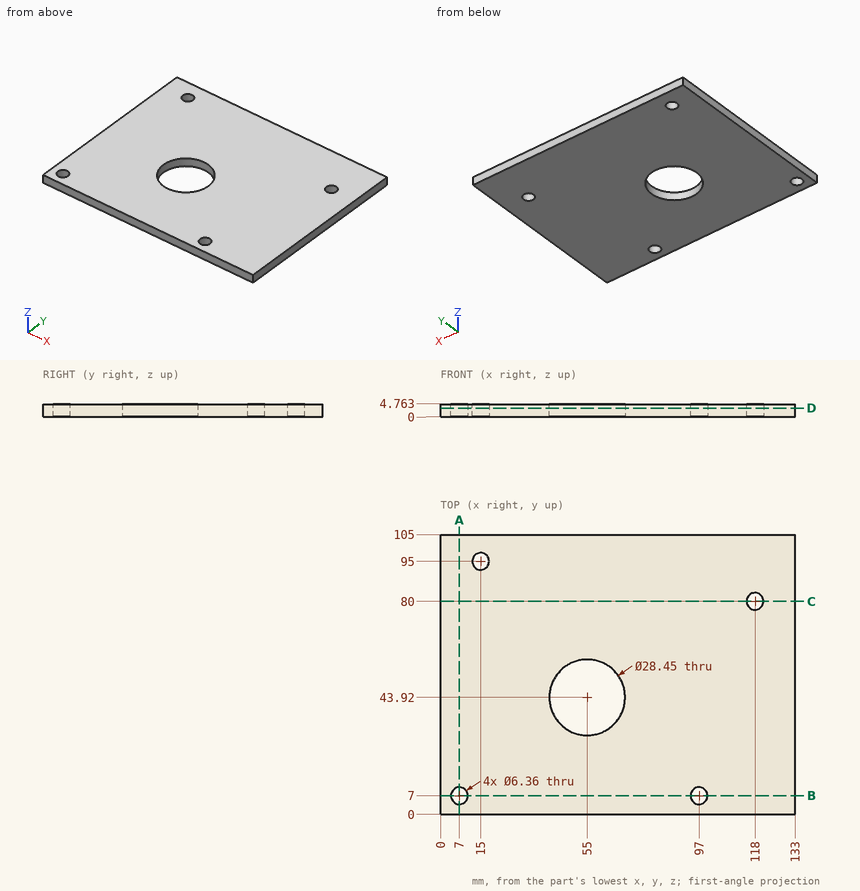
Geometry check sheet. Reference: drawing and pictorial views, mm from the part's lowest x, y, z. Give positions to 0.01 mm unless a question says otherwise; leave off trailing zeros. Order: outer loops, then holes, each group sorted by start corner. A loop starts at its lowest first (then second) coordinate and runs counter-clockwise, first axis right, second up. Notation, with made-up numbers: M -23.75,-16 L -8.75,-16 A23 ccw -8.75,19 Z; hole C 21,17 d7. An arc over 180 degrees is marked long. Answer in a Markdown table with one row per item.
1) Cross-section at A-A, the plane x = 7. Enter the section's corners in (y, z).
Filled sheet:
| item | result |
|---|---|
| outline | M 0,0 L 3.82,0 L 3.82,4.76 L 0,4.76 Z; M 10.18,0 L 105,0 L 105,4.76 L 10.18,4.76 Z |
2) Cross-section at C-C, the plane y = 80. Enter the section's corners in (x, z).
Filled sheet:
| item | result |
|---|---|
| outline | M 0,0 L 114.82,0 L 114.82,4.76 L 0,4.76 Z; M 121.18,0 L 133,0 L 133,4.76 L 121.18,4.76 Z |
3) Cross-section at B-B, the plane y = 7. Enter the section's corners in (x, z).
Filled sheet:
| item | result |
|---|---|
| outline | M 0,0 L 3.82,0 L 3.82,4.76 L 0,4.76 Z; M 10.18,0 L 93.82,0 L 93.82,4.76 L 10.18,4.76 Z; M 100.18,0 L 133,0 L 133,4.76 L 100.18,4.76 Z |
4) Thickness scan on L1, parallel to Y at x = 7, z = 2.8; L2, parallel to Y at x = 118, z = 1.6; L3, parallel to X at y = 8, z = 0.55. Record the ranges inside material, lowest first. Write a range as [from, to].
Filled sheet:
| item | result |
|---|---|
| L1 | y = [0, 3.82], [10.18, 105] |
| L2 | y = [0, 76.82], [83.18, 105] |
| L3 | x = [0, 3.98], [10.02, 93.98], [100.02, 133] |
5) Cross-section at D-D, the plane z = 3.25. Count the separate pieces of the cut face and the enclosed holes in it, plus the area to 3 significant figures.
Filled sheet:
| item | result |
|---|---|
| separate pieces | 1 |
| enclosed holes | 5 |
| area | 13,200 mm2 |
